Design review of the part built by this model. Coordinates are the model's own, in mm. A direction names the side the tool comes from. Coordinates: 2 decimals unless noted, no trailing zeros. Loops run counter-clockwise (first coordinate to the right, second up) from the corner with the lowest first, then second, coordinate; pieces in that order, holes last. Notation, with made-up numbers: M 39.5,-24 L 98.5,-24 A8 cw 98.5,-11 Z; hole C 15,11 d9. An arc over 180 degrees is marked long. Put each result on its own line as item: value. Start each with the question number.
(1) Take a section at B-B, the plane x = 35.5. Give the boundary of the cut face in (y, z), then the cut area to 3 significant figures.
(2) For faces 5 (the flat face through (20, 0, 19)), 6 (the flat face through (20, -28, 20)), 7 (the flat face through (15, -28, 1)), list the 3-axis set-ups (+Z, -Z, +X, -X, +Y, -Y) from which the entire face can be reached by the end or side of a thin tool; tool diameter is ignored.
(3) Take a section at A-A, the plane z = 23.5. Give the boundary of the cut face in (x, y), then the cut area to 3 significant figures.
(4) The part is to be moulded in two halves that separate along Z. For faces 1 (the flat face through (20, -25, 20)), 2 (the flat face through (20, -15, 0)), 3 (the flat face through (0, -15, 15)), 4 (the flat face through (11.13, -26.48, 37.92)), say which applies: +Z half, -Z half, draft (parallel to the pull), parting line (faces both ways), or undercut.
(5) Take a section at C-C, the plane y = -2.5. Give the boundary of the cut face in (x, z).
(6) For probe 1 along Y at (x, z) = (2.5, 18); probe 2 along X at (y, z) = (-25.75, 16); probe 3 along X at (y, z) = (-27.25, 31), list the stretches that pass through material, from the lowest coordinate up. Write a range as [from, to].
(7) Take a section at D-D, the plane z = 7. Give the boundary of the cut face in (x, y), then the cut area to 3 significant figures.
(8) Clearance check with flat-ended pins moving along their axes: pin 1 (2 mm diameter, centred on x = 13, z = 0.5, fed in from -Y); pin 2 (6 mm diameter, centred on y = -4.5, z = 34, fed in from -X); pin 3 (10 mm diameter, centred on x = 10, y = -22.5, fed in from +Z). State where each tip first meets the part, or that it passes through.
```python
from build123d import *

# Parameters (mm, degrees)
F1_DEPTH = 30
F2_T     = -2
F3_W     = 9.0548824519
F3_H     = 13.9939039946
F4_DEPTH = 2
F5_DEPTH = 25


with BuildPart() as f1:
    # F0 (on Front) → F1 (new body)
    with BuildSketch(Plane.XZ):
        Polygon((0, 30), (0, 0), (40, 0), (40, 30), (20, 49.2188770223), align=None)
    extrude(amount=F1_DEPTH)

    # F2 (hollow: no face is removed)
    offset(amount=F2_T, mode=Mode.SUBTRACT)

    # F3 (on face) → F4 (cut)
    with BuildSketch(Plane.XZ.offset(30)):
        with Locations((15.2286598459, 6.9969519973)):
            Rectangle(F3_W, F3_H)
    extrude(amount=-F4_DEPTH, mode=Mode.SUBTRACT)

    # F0 (on Front) → F5 (join)
    with BuildSketch(Plane.XZ):
        Polygon((0, 30), (0, 0), (40, 0), (40, 30), (20, 49.2188770223), align=None)
    extrude(amount=F5_DEPTH)


solid = f1.part
```
Computed values:
1. outline: M -30,0 L 0,0 L 0,34.32 L -30,34.32 Z; hole M -28,2 L -25,2 L -25,31.55 L -28,31.55 Z
1. area: 941 mm^2
2. face 5: +Z, -Z, +X, -X, +Y
2. face 6: none
2. face 7: -Z, -Y
3. outline: M 0,-30 L 40,-30 L 40,0 L 0,0 Z; hole M 2,-28 L 38,-28 L 38,-25 L 2,-25 Z
3. area: 1,090 mm^2
4. face 1: undercut
4. face 2: -Z half
4. face 3: draft
4. face 4: undercut
5. outline: M 0,0 L 40,0 L 40,30 L 20,49.22 L 0,30 Z
6. probe 1: y = [-30, -28], [-25, 0]
6. probe 2: x = [0, 2], [38, 40]
6. probe 3: x = [1.04, 3.93], [36.07, 38.96]
7. outline: M 0,-30 L 10.7,-30 L 10.7,-28 L 2,-28 L 2,-25 L 38,-25 L 38,-28 L 19.76,-28 L 19.76,-30 L 40,-30 L 40,0 L 0,0 Z
7. area: 1,070 mm^2
8. pin 1: stops at y = -28
8. pin 2: stops at x = 1.04
8. pin 3: stops at z = 44.41
